Verification items for the finished model (mm, model axes). A direction names the side the tool comes from. Give positions to 0.01 mm unless a question says otherwise; leave off trailing zeros. Order: outer loops, then holes, each group sorted by start corner. A loop starts at its lowest first (then second) coordinate and runs counter-clockwise, first axis right, second up. Notation, with made-up numbers: M 38,75 L 65,75 A17 cw 65,83 Z; hole C 75,-24.5 d3. An arc over 180 degrees is marked long. Answer as a JSON object with one key per item and string values.
```python
from build123d import *

# Parameters (mm, degrees)
SKETCH1_W           = 500
SKETCH1_H           = 20
SKETCH1_R           = 5
SKETCH1_R_2         = 2.5
BOSS_EXTRUDE1_DEPTH = 10
FILLET1_R           = 10
SKETCH2_R           = 5
BOSS_EXTRUDE2_DEPTH = 20
FILLET2_R           = 5


with BuildPart() as part:
    # Sketch1 → Boss-Extrude1 (new body)
    with BuildSketch(Plane.XY):
        Rectangle(SKETCH1_W, SKETCH1_H)
        with Locations((-240, 0)):
            Circle(SKETCH1_R, mode=Mode.SUBTRACT)
        with Locations((245, 0)):
            Circle(SKETCH1_R_2, mode=Mode.SUBTRACT)
    extrude(amount=BOSS_EXTRUDE1_DEPTH)

    # Fillet1
    fillet1_edges = [part.edges().sort_by_distance(p)[0] for p in [
        (250, -10, 5),
        (250, 10, 5),
        (-250, -10, 5),
        (-250, 10, 5),
    ]]
    fillet(fillet1_edges, radius=FILLET1_R - 0.0001)  # a hair under: the kernel refuses the full size

    # Sketch2 → Boss-Extrude2 (add)
    with BuildSketch(Plane(origin=(0, 0, 0), x_dir=(-1, 0, 0), z_dir=(0, 0, -1))):
        with Locations(Location((-10, 0, 0), (0, 0, 180))):
            Circle(SKETCH2_R)
    extrude(amount=BOSS_EXTRUDE2_DEPTH)

    # Fillet2
    fillet2_edges = [part.edges().sort_by_distance(p)[0] for p in [
        (5, 0, 0),
    ]]
    fillet(fillet2_edges, radius=FILLET2_R - 0.0001)  # a hair under: the kernel refuses the full size


solid = part.part
```
Q1. Section check A-A on x = 55. Record the cut outline in (y, z).
Resolved:
{"outline": "M -10,0 L 10,0 L 10,10 L -10,10 Z"}
Q2. Gauge pin test, flat ends, axial feed: pin 1 Ø8 at (y, z) = (-4.5, 1.5) entering from -X; pin 2 Ø2 at (y, z) = (-7, 0.5) entering from +X; pin 3 Ø8 at (x, y) = (-62, 3.5) entering from -Z. Record the tip position at first contact, or that the pin passes through.
Resolved:
{"pin 1": "stops at x = -249.99", "pin 2": "stops at x = 248", "pin 3": "stops at z = 0"}
Q3. Tool access check on faces 1 (the face through (-3, -10, 5)), 2 (the face through (14.77, -1.5, -12.39)). Record the directions out of +Z, -Z, +X, -X, +Y, -Y that give a thin tool (end or side, any length) a straight path to the whole face; none if there is none.
Resolved:
{"face 1": "+Z, -Z, +X, -X, -Y", "face 2": "-Z"}
Q4. Material ranges on L1, parallel to Y at x = -240, z = 5.5; L2, parallel to X at y = 1, z = 0.5; L3, parallel to X at y = -2, z = 7.25, recorded low to high.
Resolved:
{"L1": "y = -10 to -5, 5 to 10", "L2": "x = -249.95 to -244.9, -235.1 to 242.71, 247.29 to 249.95", "L3": "x = -249.8 to -244.58, -235.42 to 243.5, 246.5 to 249.8"}
